Could you check a few things on this model? Use its own coordinates, in mm. Coordinates: 2 decimals unless noted, no trailing zeros. Write each loop counter-clockwise with the first axis right and the second up, starting at its lowest first coordinate (ties: lowest second). Pieces come first, ordered by that corner, then holes.
Item 1: If I drill on probe 1 along X at (y, z) = (2.35, 80.5); probe 2 along X at (y, z) = (0.85, -76.57) (3 decimals); probe 3 along X at (y, z) = (2.55, 84.75) (3 decimals), over which ranges is the centre line in solid material (lowest first)?
Item 2: I want a section at A-A on z = -66. Please give me the cut outline in (x, y) (3 decimals).
Item 3: I want a section at C-C on z = 72. Please give me the cut outline in (x, y) (3 decimals), then the cut area to 3 significant figures.
Item 4: I want a section at B-B on y = 1. State how many separate pieces and enclosed holes the cut face has, then the cut area to 3 significant figures.
from build123d import *

# Parameters (mm, degrees)
SKETCH1_W               = 130
SKETCH1_H               = 184.5
BOSS_EXTRUDE1_DEPTH     = 3.175
SKETCH4_R               = 1.475
CUT_EXTRUDE3_DEPTH      = 113.894389254
SKETCH5_R               = 1.475
CUT_EXTRUDE4_DEPTH      = 10
SKETCH6_W               = 130
SKETCH6_H               = 3.175
BOSS_EXTRUDE2_DEPTH     = 1
CUT_EXTRUDE5_DEPTH      = 114.712985736
CUT_EXTRUDE5_DEPTH_BACK = 114.712985736
SKETCH7_W               = 6.35
SKETCH7_H               = 22
SKETCH8_W               = 65
SKETCH8_H               = 10
CUT_EXTRUDE6_DEPTH      = 10
SKETCH9_R               = 1.475
CUT_EXTRUDE7_DEPTH      = 75
SKETCH10_W              = 78.139021678
SKETCH10_H              = 97.798202291
BOSS_EXTRUDE3_DEPTH     = 3.175
SKETCH11_R              = 1.475
CUT_EXTRUDE8_DEPTH      = 10


with BuildPart() as part:
    # Sketch1 → Boss-Extrude1 (new body)
    with BuildSketch(Plane(origin=(0, 0, 0), x_dir=(1, 0, 0), z_dir=(0, 1, 0))):
        Rectangle(SKETCH1_W, SKETCH1_H)
    extrude(amount=BOSS_EXTRUDE1_DEPTH)

    # Sketch4 → Cut-Extrude3 (cut, through all)
    with BuildSketch(Plane(origin=(0, 0, 0), x_dir=(-1, 0, 0), z_dir=(0, -1, 0))):
        with Locations(Location((-57.5, -84.75, 0), (0, 0, 90))):
            Circle(SKETCH4_R)
        with Locations(Location((-57.5, -67.75, 0), (0, 0, 90))):
            Circle(SKETCH4_R)
        with Locations(Location((57.5, -84.75, 0), (0, 0, 90))):
            Circle(SKETCH4_R)
        with Locations(Location((57.5, -67.75, 0), (0, 0, 90))):
            Circle(SKETCH4_R)
        with BuildLine():
            Line((-57.35, 85.775), (-57.35, 55.775))
            ThreePointArc((-57.35, 55.775), (-58.825, 54.3), (-60.3, 55.775))
            Line((-60.3, 55.775), (-60.3, 85.775))
            ThreePointArc((-60.3, 85.775), (-58.825, 87.25), (-57.35, 85.775))
        make_face()
        with BuildLine():
            Line((60.3, 85.775), (60.3, 55.775))
            ThreePointArc((60.3, 55.775), (58.825, 54.3), (57.35, 55.775))
            Line((57.35, 55.775), (57.35, 85.775))
            ThreePointArc((57.35, 85.775), (58.825, 87.25), (60.3, 85.775))
        make_face()
    extrude(amount=-CUT_EXTRUDE3_DEPTH, mode=Mode.SUBTRACT)

    # Sketch5 → Cut-Extrude4 (cut)
    with BuildSketch(Plane.XZ):
        with Locations(Location((-24.475, -85.775, 0), (0, 0, 270))):
            Circle(SKETCH5_R)
        with Locations(Location((24.475, -85.775, 0), (0, 0, 270))):
            Circle(SKETCH5_R)
    extrude(amount=-CUT_EXTRUDE4_DEPTH, mode=Mode.SUBTRACT)

    # Sketch6 → Boss-Extrude2 (add)
    with BuildSketch(Plane(origin=(0, 0, -92.25), x_dir=(-1, 0, 0), z_dir=(0, 0, -1))):
        with Locations((0, 1.5875)):
            Rectangle(SKETCH6_W, SKETCH6_H)
    extrude(amount=BOSS_EXTRUDE2_DEPTH)

    # Sketch7 → Cut-Extrude5 (cut, two sides: drawn at the far end of the back side and taken through both)
    with BuildSketch(Plane(origin=(0, 3.175, 0), x_dir=(1, 0, 0), z_dir=(0, 1, 0)).offset(-CUT_EXTRUDE5_DEPTH_BACK)):
        with Locations((-22.175, -76.48843537)):
            Rectangle(SKETCH7_W, SKETCH7_H)
        with Locations((22.175, -76.48843537)):
            Rectangle(SKETCH7_W, SKETCH7_H)
    extrude(amount=CUT_EXTRUDE5_DEPTH + CUT_EXTRUDE5_DEPTH_BACK, mode=Mode.SUBTRACT)

    # Sketch8 → Cut-Extrude6 (cut)
    with BuildSketch(Plane.XZ):
        with Locations((0, 31.25)):
            Rectangle(SKETCH8_W, SKETCH8_H)
    extrude(amount=-CUT_EXTRUDE6_DEPTH, mode=Mode.SUBTRACT)

    # Sketch9 → Cut-Extrude7 (cut)
    with BuildSketch(Plane(origin=(0, 0, 0), x_dir=(-1, 0, 0), z_dir=(0, -1, 0))):
        with BuildLine():
            ThreePointArc((-28.525, -12.75), (-28.957017498, -11.707017498), (-30, -11.275))
            Line((-30, -11.275), (-30, -12.75))
            Line((-30, -12.75), (-28.525, -12.75))
        make_face()
        with BuildLine():
            Line((-30, -12.75), (-30, -11.275))
            ThreePointArc((-30, -11.275), (-31.042982502, -13.792982502), (-28.525, -12.75))
            Line((-28.525, -12.75), (-30, -12.75))
        make_face()
        with BuildLine():
            ThreePointArc((-30, 73.775), (-28.957017498, 74.207017498), (-28.525, 75.25))
            Line((-28.525, 75.25), (-30, 75.25))
            Line((-30, 75.25), (-30, 73.775))
        make_face()
        with BuildLine():
            Line((-30, 75.25), (-28.525, 75.25))
            ThreePointArc((-28.525, 75.25), (-31.042982502, 76.292982502), (-30, 73.775))
            Line((-30, 73.775), (-30, 75.25))
        make_face()
        with Locations(Location((30, -12.75, 0), (0, 0, 90))):
            Circle(SKETCH9_R)
        with Locations(Location((30, 75.25, 0), (0, 0, 90))):
            Circle(SKETCH9_R)
    extrude(amount=-CUT_EXTRUDE7_DEPTH, mode=Mode.SUBTRACT)

    # Sketch10 → Boss-Extrude3 (add)
    with BuildSketch(Plane(origin=(0, 0, 0), x_dir=(-1, 0, 0), z_dir=(0, -1, 0))):
        with Locations((-1.9908031, 30.735322083)):
            Rectangle(SKETCH10_W, SKETCH10_H)
    extrude(amount=-BOSS_EXTRUDE3_DEPTH)

    # Sketch11 → Cut-Extrude8 (cut)
    with BuildSketch(Plane(origin=(0, 0, 0), x_dir=(-1, 0, 0), z_dir=(0, -1, 0))):
        with Locations(Location((31.39, -19.98, 0), (0, 0, 90))):
            Circle(SKETCH11_R)
        with Locations(Location((31.39, 76.57, 0), (0, 0, 90))):
            Circle(SKETCH11_R)
        with Locations(Location((-31.39, -19.98, 0), (0, 0, 90))):
            Circle(SKETCH11_R)
        with Locations(Location((-31.39, 76.57, 0), (0, 0, 90))):
            Circle(SKETCH11_R)
    extrude(amount=-CUT_EXTRUDE8_DEPTH, mode=Mode.SUBTRACT)


solid = part.part
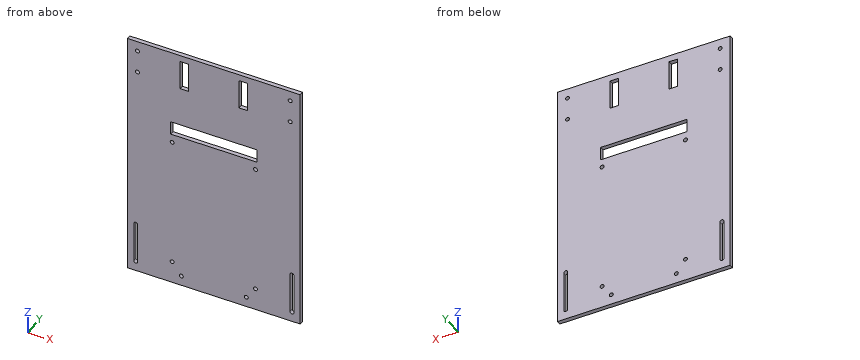
Response values:
1. probe 1: x = -65 to -25.35, -19 to 19, 25.35 to 65
1. probe 2: x = -65 to -60.3, -57.35 to -32.865, -29.915 to 29.915, 32.865 to 57.35, 60.3 to 65
1. probe 3: x = -65 to -58.975, -56.025 to -25.35, -19 to 19, 25.35 to 56.025, 58.975 to 65
2. outline: (-65, 0) - (-60.3, 0) - (-60.3, 3.175) - (-65, 3.175) - close; (-57.35, 0) - (57.35, 0) - (57.35, 3.175) - (-57.35, 3.175) - close; (60.3, 0) - (65, 0) - (65, 3.175) - (60.3, 3.175) - close
3. outline: (-65, 0) - (-25.35, 0) - (-25.35, 3.175) - (-65, 3.175) - close; (-19, 0) - (19, 0) - (19, 3.175) - (-19, 3.175) - close; (25.35, 0) - (65, 0) - (65, 3.175) - (25.35, 3.175) - close
3. area: 372 mm2
4. separate pieces: 1
4. enclosed holes: 15
4. area: 22,900 mm2
